Verification items for the finished model (mm, model axes). A direction names the side the tool comes from. Round coordinates to 2 decimals unless told otherwise and drop trailing zeros. Order: outer loops, then holes, each group sorted by start corner. A loop starts at its lowest first (then second) coordinate and runs counter-clockwise, first axis right, second up. Notation, with made-up numbers: (7.5, 80.25) -> (36.5, 80.25) arc R11 ccw to (36.5, 85.25) -> close; hole circle Ø2 at (62, -3.75). An arc over 180 degrees is marked (long way). Put each result on its own line as item: value.
```python
from build123d import *

# Parameters (mm, degrees)
ESQUISSE1_R             = 4.25
ESQUISSE1_R_2           = 1.5
BOSS_EXTRU_1_DEPTH      = 5
ESQUISSE2_R             = 1.5
ESQUISSE2_R_2           = 1.6
BOSS_EXTRU_2_DEPTH      = 5
CONG_1_R                = 1
ENL_V_MAT_EXTRU_1_DEPTH = 10.5
CONG_2_R                = 5


with BuildPart() as part:
    # Esquisse1 → Boss.-Extru.1 (new body)
    with BuildSketch(Plane.XY):
        with BuildLine():
            Line((30.5, 0), (30.5, 3))
            ThreePointArc((30.5, 3), (29.035533906, 6.535533906), (25.5, 8))
            Line((25.5, 8), (22.5, 8))
            Line((22.5, 8), (18.5, 12))
            Line((18.5, 12), (-26.5, 12))
            Line((-26.5, 12), (-30.5, 8))
            Line((-30.5, 8), (-30.5, 0))
            Line((-30.5, 0), (-30.5, -8))
            Line((-30.5, -8), (-26.5, -12))
            Line((-26.5, -12), (18.5, -12))
            Line((18.5, -12), (22.5, -8))
            Line((22.5, -8), (25.5, -8))
            ThreePointArc((25.5, -8), (29.035533906, -6.535533906), (30.5, -3))
            Line((30.5, -3), (30.5, 0))
        make_face()
        with Locations((-16.5, 0)):
            Circle(ESQUISSE1_R, mode=Mode.SUBTRACT)
        with Locations((-7.5, -8.5)):
            Circle(ESQUISSE1_R_2, mode=Mode.SUBTRACT)
        with Locations((8.5, 0)):
            Circle(ESQUISSE1_R, mode=Mode.SUBTRACT)
        with Locations((-7.5, 8.5)):
            Circle(ESQUISSE1_R_2, mode=Mode.SUBTRACT)
        with Locations((26.5, 4)):
            Circle(ESQUISSE1_R_2, mode=Mode.SUBTRACT)
        with Locations((26.5, -4)):
            Circle(ESQUISSE1_R_2, mode=Mode.SUBTRACT)
    extrude(amount=BOSS_EXTRU_1_DEPTH)

    # Esquisse2 → Boss.-Extru.2 (add)
    with BuildSketch(Plane(origin=(0, 0, 0), x_dir=(-1, 0, 0), z_dir=(0, 0, -1))):
        with BuildLine():
            Line((-30.5, 17), (-30.5, 8))
            Line((-30.5, 8), (-25.5, 8))
            ThreePointArc((-25.5, 8), (-29.035533906, 6.535533906), (-30.5, 3))
            Line((-30.5, 3), (-30.5, -3))
            ThreePointArc((-30.5, -3), (-29.035533906, -6.535533906), (-25.5, -8))
            Line((-25.5, -8), (-30.5, -8))
            Line((-30.5, -8), (-30.5, -16))
            Line((-30.5, -16), (-30.5, -17))
            Line((-30.5, -17), (-36.257359313, -17))
            Line((-36.257359313, -17), (-36.257359313, -21))
            ThreePointArc((-36.257359313, -21), (-40.5, -24), (-44.742640687, -21))
            Line((-44.742640687, -21), (-44.742640687, -17))
            Line((-44.742640687, -17), (-50.5, -17))
            Line((-50.5, -17), (-50.5, 17))
            Line((-50.5, 17), (-44.742640687, 17))
            Line((-44.742640687, 17), (-44.742640687, 21))
            ThreePointArc((-44.742640687, 21), (-40.5, 24), (-36.257359313, 21))
            Line((-36.257359313, 21), (-36.257359313, 17))
            Line((-36.257359313, 17), (-30.5, 17))
        make_face()
        with Locations((-40.5, 13.5)):
            Circle(ESQUISSE2_R, mode=Mode.SUBTRACT)
        with Locations((-40.5, -13.5)):
            Circle(ESQUISSE2_R, mode=Mode.SUBTRACT)
        with Locations((-40.5, 19.5)):
            Circle(ESQUISSE2_R_2, mode=Mode.SUBTRACT)
        with Locations((-40.5, -19.5)):
            Circle(ESQUISSE2_R_2, mode=Mode.SUBTRACT)
    extrude(amount=-BOSS_EXTRU_2_DEPTH)

    # Congé1
    cong_1_edges = [part.edges().sort_by_distance(p)[0] for p in [
        (44.742640687, -21, 2.5),
    ]]
    fillet(cong_1_edges, radius=CONG_1_R)

    # Esquisse5 → Enlèv. mat.-Extru.1 (cut)
    with BuildSketch(Plane.XY.offset(5)):
        with BuildLine():
            Line((37.257359313, 17), (37.257359313, 19.5))
            ThreePointArc((37.257359313, 19.5), (40.5, 22.742640687), (43.742640687, 19.5))
            Line((43.742640687, 19.5), (43.742640687, 17))
            Line((43.742640687, 17), (46.702112937, 17))
            Line((46.702112937, 17), (46.702112937, 27.914494418))
            Line((46.702112937, 27.914494418), (36.257359313, 27.914494418))
            Line((36.257359313, 27.914494418), (36.257359313, 17))
            Line((36.257359313, 17), (37.257359313, 17))
        make_face()
        with BuildLine():
            Line((43.742640687, -19.5), (43.742640687, -17))
            Line((43.742640687, -17), (44.742640687, -17))
            Line((44.742640687, -17), (44.742640687, -31.949987741))
            Line((44.742640687, -31.949987741), (43.742640687, -31.949987741))
            Line((43.742640687, -31.949987741), (37.257359313, -31.949987741))
            Line((37.257359313, -31.949987741), (34.849139441, -17))
            Line((34.849139441, -17), (37.257359313, -17))
            Line((37.257359313, -17), (37.257359313, -19.5))
            ThreePointArc((37.257359313, -19.5), (40.5, -22.742640687), (43.742640687, -19.5))
        make_face()
    extrude(amount=-ENL_V_MAT_EXTRU_1_DEPTH, mode=Mode.SUBTRACT)

    # Congé2
    cong_2_edges = [part.edges().sort_by_distance(p)[0] for p in [
        (22.5, -8, 2.5),
        (22.5, 8, 2.5),
        (30.5, 8, 2.5),
        (30.5, -8, 2.5),
    ]]
    fillet(cong_2_edges, radius=CONG_2_R)


solid = part.part
```
Item 1: Sectioned sample at C-C, the plane y = 0. Record the boundary of the cut face in (x, z), then the cut area to 3 significant figures.
Geometry check:
outline: (-30.5, 0) -> (-20.75, 0) -> (-20.75, 5) -> (-30.5, 5) -> close; (-12.25, 0) -> (4.25, 0) -> (4.25, 5) -> (-12.25, 5) -> close; (12.75, 0) -> (50.5, 0) -> (50.5, 5) -> (12.75, 5) -> close
area: 320 mm2
Item 2: Material ranges on line 1 along Y through (x, z) = (-7.5, 2.8); line 2 along Y through (x, z) = (40.5, 3.35); line 3 along Y through (x, z) = (-16.5, 2.2), recorded low to high.
Geometry check:
line 1: -12 to -10, -7 to 7, 10 to 12
line 2: -22.74 to -21.1, -17.9 to -15, -12 to 12, 15 to 17.9, 21.1 to 22.74
line 3: -12 to -4.25, 4.25 to 12
Item 3: Tool access check on faces 4 (the face through (30.5, 15, 2)), 5 (the face through (22.68, -8.37, 2.54)), 6 (the face through (30.5, -15, 2)), 7 (the face through (43.743, 18, 3)). Record the directions out of +Z, -Z, +X, -X, +Y, -Y that give a thin tool (end or side, any length) a straight path to the whole face; none if there is none.
Geometry check:
face 4: +Z, -Z, -X, +Y
face 5: +Z, -Z, -Y
face 6: +Z, -Z, -X, -Y
face 7: +Z, -Z, +X, +Y
Item 4: Sectioned sample at A-A, the plane x = -16.5. Record the boundary of the cut face in (y, z), then the cut area to 3 significant figures.
Geometry check:
outline: (-12, 0) -> (-4.25, 0) -> (-4.25, 5) -> (-12, 5) -> close; (4.25, 0) -> (12, 0) -> (12, 5) -> (4.25, 5) -> close
area: 77.5 mm2
Item 5: Sectioned sample at D-D, the plane x = 40.5. Record the boundary of the cut face in (y, z), then the cut area to 3 significant figures.
Geometry check:
outline: (-22.74, 0) -> (-21.1, 0) -> (-21.1, 5) -> (-22.74, 5) -> close; (-17.9, 0) -> (-15, 0) -> (-15, 5) -> (-17.9, 5) -> close; (-12, 0) -> (12, 0) -> (12, 5) -> (-12, 5) -> close; (15, 0) -> (17.9, 0) -> (17.9, 5) -> (15, 5) -> close; (21.1, 0) -> (22.74, 0) -> (22.74, 5) -> (21.1, 5) -> close
area: 165 mm2
Item 6: Sectioned sample at B-B, the plane x = -7.5. Record the boundary of the cut face in (y, z), then the cut area to 3 significant figures.
Geometry check:
outline: (-12, 0) -> (-10, 0) -> (-10, 5) -> (-12, 5) -> close; (-7, 0) -> (7, 0) -> (7, 5) -> (-7, 5) -> close; (10, 0) -> (12, 0) -> (12, 5) -> (10, 5) -> close
area: 90.0 mm2
Item 7: Depth check by flat-ended pin: pin 1 Ø1.2 at (y, z) = (14.5, 3) entering from -X; pin 2 Ø2.5 at (x, y) = (40.5, 13.5) entering from +Z; pin 3 Ø0.8 at (y, z) = (18.5, 2.5) entering from -X; pin 4 Ø3 at (x, z) = (10.5, 4) entering from -Y. Enter the tip coordinate at first touch or a pass-through.
Geometry check:
pin 1: x = 30.5
pin 2: through
pin 3: x = 37.26
pin 4: y = -12
Item 8: Release check for a two-part mould opening along Y. For faces 1 (the face through (50.5, 0, 2)), 2 (the face through (47, 17, 3)), 3 (the face through (4.254, 0.187, 2.465)) record: pulls with the +Y half, pulls with the -Y half, needs draft (parallel to the pull), parting line crosses it, or undercut.
Geometry check:
face 1: needs draft
face 2: pulls with the +Y half
face 3: undercut
